The listing builds one solid part. Answer for the finished solid, in the listing's coordinates (mm). Face numbers are marked on the shaded views. A direction names the side the tool comes from. Round coordinates to 2 decimals unless told otherwise and drop trailing zeros. Write each loop counter-clockwise with the first axis right and the second up, starting at its lowest first coordinate (ties: lowest second). Pieces come first, ordered by that corner, then holes.
(1) Each of these flat-tipped pins is pushed along its axis until it touches: pin 1 Ø10 at (y, z) = (21.5, 4.5) entering from +X; pin 2 Ø4 at (x, z) = (-7, -25) entering from -Y; pin 3 Ø8 at (y, z) = (16.5, -14) entering from -X; pin 4 Ø8 at (y, z) = (25.5, -23) entering from -X. Where does it stop, or does it pass through?
(2) The mould has two halves that part along X. Classify the marked faces 1, 2 and 3: +X half, -X half, draft (parallel to the pull), parting line (faces both ways), or undercut.
(3) A cutting plane is placed at A-A, the plane y = 12. Give the vertices of the cut face in (x, z).
(4) For the marked faces 4, 5 and 6, determine the directions among +Z, -Z, +X, -X, +Y, -Y from which every point of the face is accessible in a straight line to the end or side of a thin tool.
(5) A cutting plane is placed at B-B, the plane z = -27. Give the vertices of the cut face in (x, y), and give its area (3 significant figures).
(6) A cutting plane is placed at C-C, the plane x = -5. Give the vertices of the cut face in (y, z).
(7) Find the intervals of material crossed by probe 1 along X at (y, z) = (0.8, -25); probe 2 along Z at (x, y) = (-7, 2.35); probe 3 along X at (y, z) = (1.75, -25), in increasing order.
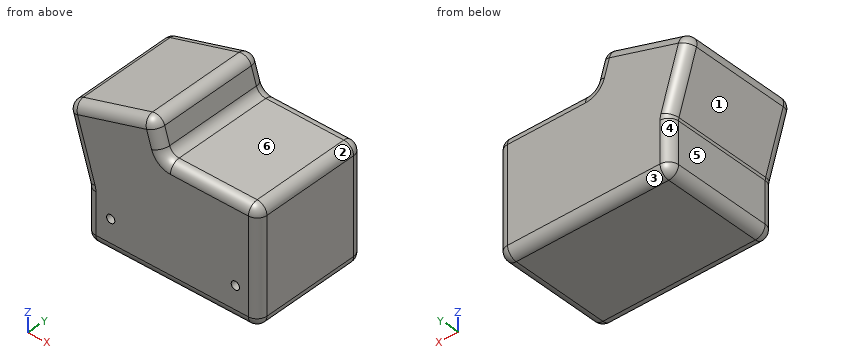
from build123d import *

# Parameters (mm, degrees)
BOSS_EXTRUDE1_DEPTH             = 36
FILLET1_R                       = 3
TAP_DRILL_FOR_M3X0_5_TAP1_D     = 2.5
TAP_DRILL_FOR_M3X0_5_TAP1_DEPTH = 3
TAP_DRILL_FOR_M3X0_5_TAP1_TIP   = 0.751075774


with BuildPart() as part:
    # Sketch1 → Boss-Extrude1 (new body)
    with BuildSketch(Plane(origin=(0, 0, 0), x_dir=(1, 0, 0), z_dir=(0, 1, 0))):
        with BuildLine():
            Line((0, 3), (0, 32))
            ThreePointArc((0, 32), (-0.878679656, 34.121320344), (-3, 35))
            Line((-3, 35), (-49.5, 35))
            ThreePointArc((-49.5, 35), (-51.621320344, 34.121320344), (-52.5, 32))
            Line((-52.5, 32), (-52.5, 19.444534932))
            ThreePointArc((-52.5, 19.444534932), (-52.53240259, 19.004801361), (-52.628910409, 18.574566795))
            Line((-52.628910409, 18.574566795), (-57.971756527, 0.941978638))
            ThreePointArc((-57.971756527, 0.941978638), (-57.745994224, -1.34299605), (-55.970635073, -2.799079091))
            Line((-55.970635073, -2.799079091), (-34.915978072, -9.178845431))
            ThreePointArc((-34.915978072, -9.178845431), (-32.631003385, -8.953083129), (-31.174920343, -7.177723978))
            Line((-31.174920343, -7.177723978), (-29.645420421, -2.130031863))
            ThreePointArc((-29.645420421, -2.130031863), (-28.561800492, -0.590653158), (-26.77433083, 0))
            Line((-26.77433083, 0), (-3, 0))
            ThreePointArc((-3, 0), (-0.878679656, 0.878679656), (0, 3))
        make_face()
    extrude(amount=BOSS_EXTRUDE1_DEPTH)

    # Fillet1
    fillet1_edges = [part.edges().sort_by_distance(p)[0] for p in [
        (-0.878679656, 36, -34.121320344),
        (-14.887165415, 0, 0),
        (-28.561800492, 0, 0.590653158),
        (-26.25, 36, -35),
        (-30.410170382, 0, 4.65387792),
        (-32.631003385, 0, 8.953083129),
        (-45.443306572, 0, 5.988962261),
        (-57.745994224, 0, 1.34299605),
        (-55.300333468, 0, -9.758272716),
        (-52.53240259, 0, -19.004801361),
        (-52.5, 0, -25.722267466),
        (-51.621320344, 36, -34.121320344),
        (-51.621320344, 0, -34.121320344),
        (-26.25, 0, -35),
        (-0.878679656, 0, -34.121320344),
        (0, 0, -17.5),
        (-0.878679656, 0, -0.878679656),
        (-52.5, 36, -25.722267466),
        (-52.53240259, 36, -19.004801361),
        (-55.300333468, 36, -9.758272716),
        (-57.745994224, 36, 1.34299605),
        (-45.443306572, 36, 5.988962261),
        (-32.631003385, 36, 8.953083129),
        (-30.410170382, 36, 4.65387792),
        (-0.878679656, 36, -0.878679656),
        (-28.561800492, 36, 0.590653158),
        (-14.887165415, 36, 0),
        (0, 36, -17.5),
    ]]
    fillet(fillet1_edges, radius=FILLET1_R)

    # Tap Drill for M3x0.5 Tap1
    with Locations(Plane(origin=(0, 0, 0), x_dir=(-1, 0, 0), z_dir=(0, -1, 0))):
        with Locations((7, 25), (45, 25)):
            Hole(TAP_DRILL_FOR_M3X0_5_TAP1_D / 2, depth=TAP_DRILL_FOR_M3X0_5_TAP1_DEPTH)
            with Locations((0, 0, -(TAP_DRILL_FOR_M3X0_5_TAP1_DEPTH + TAP_DRILL_FOR_M3X0_5_TAP1_TIP / 2))):  # 118° drill point
                Cone(0, TAP_DRILL_FOR_M3X0_5_TAP1_D / 2, TAP_DRILL_FOR_M3X0_5_TAP1_TIP, mode=Mode.SUBTRACT)


solid = part.part
Solutions:
1. pin 1: stops at x = -1.34
1. pin 2: stops at y = 0
1. pin 3: stops at x = -55.23
1. pin 4: stops at x = -52.53
2. face 1: -X half
2. face 2: +X half
2. face 3: draft
3. outline: (-57.97, -0.94) - (-52.63, -18.57) arc R3 cw to (-52.5, -19.44) - (-52.5, -32) arc R3 ccw to (-49.5, -35) - (-3, -35) arc R3 ccw to (0, -32) - (0, -3) arc R3 ccw to (-3, 0) - (-26.77, 0) arc R3 cw to (-29.65, 2.13) - (-31.17, 7.18) arc R3 ccw to (-34.92, 9.18) - (-55.97, 2.8) arc R3 ccw to start
4. face 4: -Z, -X, +Y
4. face 5: -Z, -X, +Y, -Y
4. face 6: +Z, +X, +Y, -Y
5. outline: (-52.5, 3) arc R3 ccw to (-49.5, 0) - (-3, 0) arc R3 ccw to (0, 3) - (0, 33) arc R3 ccw to (-3, 36) - (-49.5, 36) arc R3 ccw to (-52.5, 33) - close
5. area: 1,880 mm2
6. outline: (0, -32) arc R3 ccw to (3, -35) - (33, -35) arc R3 ccw to (36, -32) - (36, -3) arc R3 ccw to (33, 0) - (3, 0) arc R3 ccw to (0, -3) - close
7. probe 1: x = -51.54 to -46.25, -43.75 to -8.25, -5.75 to -0.96
7. probe 2: z = -34.93 to -26.25, -23.75 to -0.07
7. probe 3: x = -52.23 to -46.25, -43.75 to -8.25, -5.75 to -0.27
